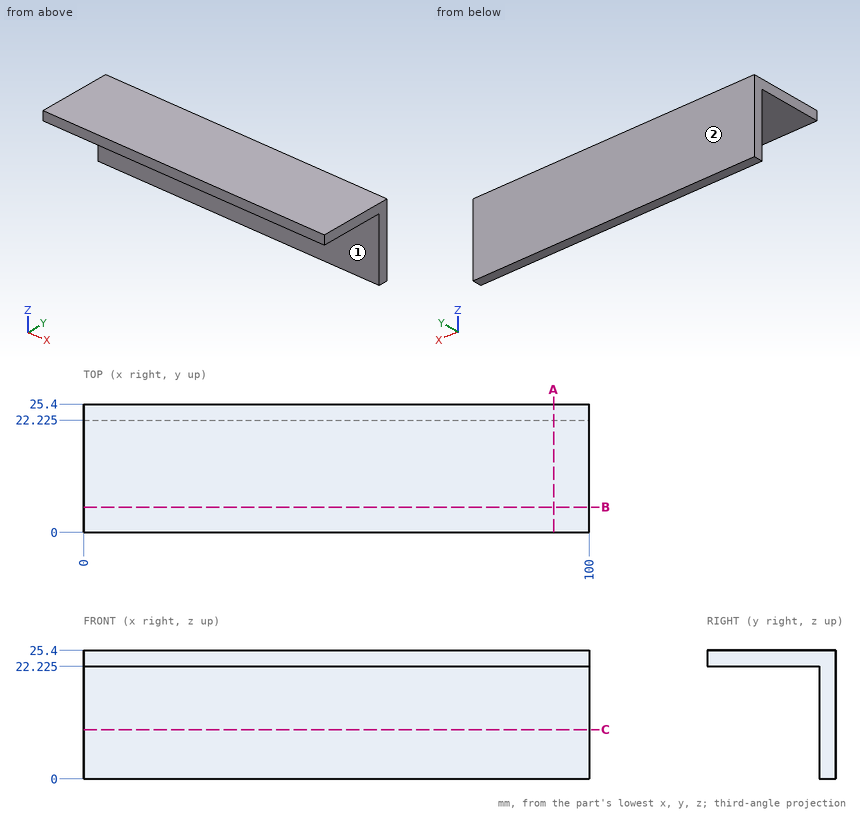
Part print with two shaded views. Sizes in mm from the minimum x, y, z corner. A direction names the side the tool comes from. Round coordinates to 2 decimals unless told otherwise and drop trailing zeros. Order: outer loops, then holes, each group sorted by start corner. A loop starts at its lowest first (then second) coordinate and runs counter-clockwise, first axis right, second up. Notation, with made-up numbers: (64.25, 70) -> (86.25, 70) arc R18 ccw to (86.25, 103) -> close; hole circle Ø4 at (87.5, 65.5). An arc over 180 degrees is marked (long way). One line per question, with ' | ' between items.
Q1. Slice it at B-B (y = 5). Write the cut outline in (x, z) (3 decimals), then the cut area to 4 significant figures.
Completed:
outline: (0, 22.225) -> (100, 22.225) -> (100, 25.4) -> (0, 25.4) -> close | area: 317.5 mm^2
Q2. Which spindle directions (+Z, -Z, +X, -X, +Y, -Y) get a long thin tool onto all of the face, cutting with end or side? Do the marked faces 1 and 2. Say none if no direction does.
Completed:
face 1: -Z, +X, -X, -Y | face 2: +Z, -Z, +X, -X, +Y
Q3. Probe probe 1 along Z at (x, y) = (66, 2) (3 decimals). List the from-to ranges inside material, lowest first.
Completed:
probe 1: z = 22.225 to 25.4
Q4. Slice it at A-A (x = 93). Write the cut outline in (y, z) (3 decimals), then the cut area to 3 significant figures.
Completed:
outline: (0, 22.225) -> (22.225, 22.225) -> (22.225, 0) -> (25.4, 0) -> (25.4, 25.4) -> (0, 25.4) -> close | area: 151 mm^2
Q5. Drop flat-ended pins along their axis: pin 1 (1 mm diameter, centred on x = 14, z = 14.5, fed in from -Y) (3 decimals); pin 2 (5 mm diameter, centred on x = 53.5, y = 20, fed in from -Z); pin 3 (8 mm diameter, centred on x = 34, y = 14, fed in from -Z) (3 decimals). Give the stop position or say it passes through.
Completed:
pin 1: stops at y = 22.225 | pin 2: stops at z = 0 | pin 3: stops at z = 22.225
